Verification items for the finished model (mm, model axes). Give positions to 0.01 mm unless a question says otherwise; leave off trailing zeros. Loops run counter-clockwise (first coordinate to the right, second up) from the corner with the lowest first, then second, coordinate; pieces in that order, holes last. Notation, with made-up numbers: (0.25, 19) - (29.25, 19) arc R13 cw to (29.25, 32) - close; hole circle Ø4 at (82.25, 2). An arc over 180 degrees is marked (long way). Put each result on its own line as item: value. Start each with the question number.
```python
from build123d import *

# Parameters (mm, degrees)
F0_R     = 4.758249
F1_DEPTH = 12.7


with BuildPart() as f1:
    # F0 (on Front) → F1 (new body)
    with BuildSketch(Plane.XZ):
        Polygon((-48.298843, 57.15), (-73.698843, 57.15), (-73.698843, -19.05), (78.701157, -19.05), (78.701157, 57.15), (53.301157, 57.15), (53.301157, 31.730622), (24.726157, 31.730622), (24.726157, 57.130622), (-21.311343, 57.237761), (-21.311343, 31.75), (-48.298843, 31.75), align=None)
        with Locations((-54.648843, 0)):
            Circle(F0_R, mode=Mode.SUBTRACT)
    extrude(amount=F1_DEPTH)


solid = f1.part
```
1) Depth check by flat-ended pin: P1, Ø4, axis at x = -64, y = -9.5, coming from the +Z side; P2, Ø1, axis at x = -39.5, y = -1.5, coming from the +Z side; P3, Ø6.5, axis at x = 40.5, y = -4, coming from the +Z side. Enter the tip coordinate at first touch or a pass-through.
2) Section check A-A, the plane z = 0. Enter the section's corners in (x, y), plus the area to 3 significant figures.
3) Section check B-B, the plane z = 39. Enter the section's corners in (x, y).
4) Draft check along X on faces 1 (the face through (-73.699, -6, 20)), 2 (the face through (-35, -6, 31.75)), 3 (the face through (-48.299, -6, 44)), 4 (the face through (1, -6, -19.05)). Enter one of: pulls with the +X half, pulls with the -X half, needs draft (parallel to the pull), parting line crosses it, or undercut.
5) Scan lines: line 1 along X through (y, z) = (-5.5, 51.5); line 2 along Z through (x, y) = (-64, -10.5); line 3 along Z through (x, y) = (-54.5, -9.75). Record each from-to range of solid material in increasing order. Write a range as from..to.
6) Section check C-C, the plane y = -9.75. Enter the section's corners in (x, z).
Results are:
1. P1: stops at z = 57.15
1. P2: stops at z = 31.75
1. P3: stops at z = 31.73
2. outline: (-73.7, -12.7) - (-59.41, -12.7) - (-59.41, 0) - (-73.7, 0) - close; (-49.89, -12.7) - (78.7, -12.7) - (78.7, 0) - (-49.89, 0) - close
2. area: 1,810 mm2
3. outline: (-73.7, -12.7) - (-48.3, -12.7) - (-48.3, 0) - (-73.7, 0) - close; (-21.31, -12.7) - (24.73, -12.7) - (24.73, 0) - (-21.31, 0) - close; (53.3, -12.7) - (78.7, -12.7) - (78.7, 0) - (53.3, 0) - close
4. face 1: pulls with the -X half
4. face 2: undercut
4. face 3: undercut
4. face 4: needs draft
5. line 1: x = -73.7..-48.3, -21.31..24.73, 53.3..78.7
5. line 2: z = -19.05..57.15
5. line 3: z = -19.05..-4.76, 4.76..57.15
6. outline: (-73.7, -19.05) - (78.7, -19.05) - (78.7, 57.15) - (53.3, 57.15) - (53.3, 31.73) - (24.73, 31.73) - (24.73, 57.13) - (-21.31, 57.24) - (-21.31, 31.75) - (-48.3, 31.75) - (-48.3, 57.15) - (-73.7, 57.15) - close; hole circle Ø9.52 at (-54.65, 0)
